For this review, take the finished solid that the model builds, in its own axes (mm). Round coordinates to 2 decimals unless told otherwise and drop trailing zeros. Order: outer loops, then holes, each group sorted by start corner. A loop starts at its lowest first (then second) coordinate and runs counter-clockwise, first axis right, second up.
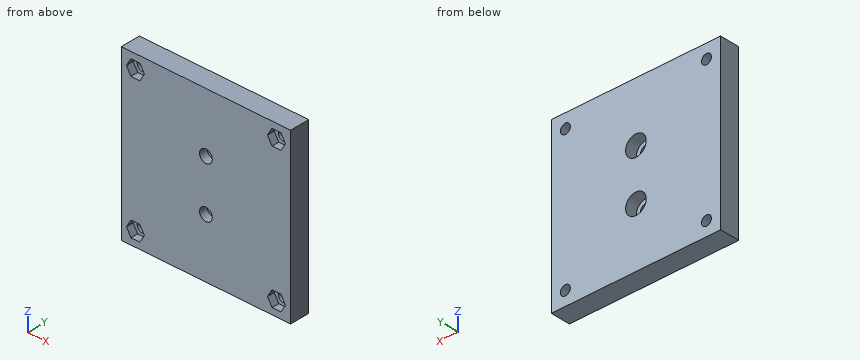
```python
from build123d import *

# Parameters (mm, degrees)
SKETCH_2_W          = 60
SKETCH_2_H          = 60
EXTRUDE_1_DEPTH     = 7
CUT_EXTRUDE_1_DEPTH = 2.6
CUT_EXTRUDE_2_REACH = 9
SKETCH_4_R          = 1.75
SKETCH_5_R          = 3.65
CUT_EXTRUDE_3_DEPTH = 4.1
CUT_EXTRUDE_4_REACH = 4.9
SKETCH_6_R          = 2.25


with BuildPart() as part:
    # 草圖2 → 填料-伸長1 (new body)
    with BuildSketch(Plane(origin=(0, 0, 0), x_dir=(1, 0, 0), z_dir=(0, 1, 0))):
        Rectangle(SKETCH_2_W, SKETCH_2_H)
    extrude(amount=EXTRUDE_1_DEPTH)

    # 草圖3 → 除料-伸長1 (cut)
    with BuildSketch(Plane.XZ):
        Polygon((-21.824573519, 25), (-23.41228676, 27.75), (-26.58771324, 27.75), (-28.175426481, 25), (-26.58771324, 22.25), (-23.41228676, 22.25), align=None)
        Polygon((23.41228676, 22.25), (21.824573519, 25), (23.41228676, 27.75), (26.58771324, 27.75), (28.175426481, 25), (26.58771324, 22.25), align=None)
        Polygon((21.824573519, -25), (23.41228676, -27.75), (26.58771324, -27.75), (28.175426481, -25), (26.58771324, -22.25), (23.41228676, -22.25), align=None)
        Polygon((-23.41228676, -22.25), (-21.824573519, -25), (-23.41228676, -27.75), (-26.58771324, -27.75), (-28.175426481, -25), (-26.58771324, -22.25), align=None)
    extrude(amount=-CUT_EXTRUDE_1_DEPTH, mode=Mode.SUBTRACT)

    # 草圖4 → 除料-伸長2 (cut, up to next)
    with BuildSketch(Plane(origin=(0, 7, 0), x_dir=(1, 0, 0), z_dir=(0, 1, 0)), mode=Mode.PRIVATE) as cut_extrude_2_sk1:
        with Locations((-25, 25)):
            Circle(SKETCH_4_R)
    cut_extrude_2_tool1 = extrude(cut_extrude_2_sk1.sketch, amount=-CUT_EXTRUDE_2_REACH, mode=Mode.PRIVATE) & part.part
    add(cut_extrude_2_tool1.solids().sort_by_distance((-25, 7, -25))[0], mode=Mode.SUBTRACT)
    # 草圖4 → 除料-伸長2 (cut, up to next)
    with BuildSketch(Plane(origin=(0, 7, 0), x_dir=(1, 0, 0), z_dir=(0, 1, 0)), mode=Mode.PRIVATE) as cut_extrude_2_sk2:
        with Locations((25, 25)):
            Circle(SKETCH_4_R)
    cut_extrude_2_tool2 = extrude(cut_extrude_2_sk2.sketch, amount=-CUT_EXTRUDE_2_REACH, mode=Mode.PRIVATE) & part.part
    add(cut_extrude_2_tool2.solids().sort_by_distance((25, 7, -25))[0], mode=Mode.SUBTRACT)
    # 草圖4 → 除料-伸長2 (cut, up to next)
    with BuildSketch(Plane(origin=(0, 7, 0), x_dir=(1, 0, 0), z_dir=(0, 1, 0)), mode=Mode.PRIVATE) as cut_extrude_2_sk3:
        with Locations((25, -25)):
            Circle(SKETCH_4_R)
    cut_extrude_2_tool3 = extrude(cut_extrude_2_sk3.sketch, amount=-CUT_EXTRUDE_2_REACH, mode=Mode.PRIVATE) & part.part
    add(cut_extrude_2_tool3.solids().sort_by_distance((25, 7, 25))[0], mode=Mode.SUBTRACT)
    # 草圖4 → 除料-伸長2 (cut, up to next)
    with BuildSketch(Plane(origin=(0, 7, 0), x_dir=(1, 0, 0), z_dir=(0, 1, 0)), mode=Mode.PRIVATE) as cut_extrude_2_sk4:
        with Locations((-25, -25)):
            Circle(SKETCH_4_R)
    cut_extrude_2_tool4 = extrude(cut_extrude_2_sk4.sketch, amount=-CUT_EXTRUDE_2_REACH, mode=Mode.PRIVATE) & part.part
    add(cut_extrude_2_tool4.solids().sort_by_distance((-25, 7, 25))[0], mode=Mode.SUBTRACT)

    # 草圖5 → 除料-伸長3 (cut)
    with BuildSketch(Plane(origin=(0, 7, 0), x_dir=(1, 0, 0), z_dir=(0, 1, 0))):
        with Locations((0, 9)):
            Circle(SKETCH_5_R)
        with Locations((0, -9)):
            Circle(SKETCH_5_R)
    extrude(amount=-CUT_EXTRUDE_3_DEPTH, mode=Mode.SUBTRACT)

    # 草圖6 → 除料-伸長4 (cut, up to next)
    with BuildSketch(Plane(origin=(0, 2.9, 0), x_dir=(1, 0, 0), z_dir=(0, 1, 0)), mode=Mode.PRIVATE) as cut_extrude_4_sk1:
        with Locations((0, 9)):
            Circle(SKETCH_6_R)
    cut_extrude_4_tool1 = extrude(cut_extrude_4_sk1.sketch, amount=-CUT_EXTRUDE_4_REACH, mode=Mode.PRIVATE) & part.part
    add(cut_extrude_4_tool1.solids().sort_by_distance((0, 2.9, -9))[0], mode=Mode.SUBTRACT)
    # 草圖6 → 除料-伸長4 (cut, up to next)
    with BuildSketch(Plane(origin=(0, 2.9, 0), x_dir=(1, 0, 0), z_dir=(0, 1, 0)), mode=Mode.PRIVATE) as cut_extrude_4_sk2:
        with Locations((0, -9)):
            Circle(SKETCH_6_R)
    cut_extrude_4_tool2 = extrude(cut_extrude_4_sk2.sketch, amount=-CUT_EXTRUDE_4_REACH, mode=Mode.PRIVATE) & part.part
    add(cut_extrude_4_tool2.solids().sort_by_distance((0, 2.9, 9))[0], mode=Mode.SUBTRACT)


solid = part.part
```
Q1. Take a section at C-C, the plane y = 4. State the section outline as (x, z) points, plus the area to 3 significant figures.
Q2. Take a section at B-B, the plane x = 0. State the section outline as (y, z) points.
Q3. Clearance check with flat-ended pins moving along their axes: pin 1 (3 mm diameter, centred on x = -25, z = -25.5, fed in from -Y); pin 2 (3 mm diameter, centred on x = 25, z = 25, fed in from +Y); pin 3 (6 mm diameter, centred on x = 0, z = 9, fed in from +Y). State where each tip first meets the part, or that it passes through.
Q4. Wall thickness on line 1 (Z direction, x = 0, y = 1.7); line 2 (X direction, y = 4.05, z = 25): over which ranges is each line inside the solid? List them lowest first.
Q5. Take a section at D-D, the plane x = -25. State the section outline as (y, z) points.
Q6. Take a section at A-A, the plane z = -9. State the section outline as (x, y) points.
Working result:
1. outline: (-30, -30) - (30, -30) - (30, 30) - (-30, 30) - close; hole circle Ø3.5 at (-25, -25); hole circle Ø3.5 at (-25, 25); hole circle Ø7.3 at (0, -9); hole circle Ø7.3 at (0, 9); hole circle Ø3.5 at (25, -25); hole circle Ø3.5 at (25, 25)
1. area: 3,480 mm2
2. outline: (0, -30) - (7, -30) - (7, -12.65) - (2.9, -12.65) - (2.9, -11.25) - (0, -11.25) - close; (0, -6.75) - (2.9, -6.75) - (2.9, -5.35) - (7, -5.35) - (7, 5.35) - (2.9, 5.35) - (2.9, 6.75) - (0, 6.75) - close; (0, 11.25) - (2.9, 11.25) - (2.9, 12.65) - (7, 12.65) - (7, 30) - (0, 30) - close
3. pin 1: stops at y = 2.6
3. pin 2: passes through
3. pin 3: stops at y = 2.9
4. line 1: z = -30 to -11.25, -6.75 to 6.75, 11.25 to 30
4. line 2: x = -30 to -26.75, -23.25 to 23.25, 26.75 to 30
5. outline: (0, -30) - (7, -30) - (7, -26.75) - (2.6, -26.75) - (2.6, -27.75) - (0, -27.75) - close; (0, -22.25) - (2.6, -22.25) - (2.6, -23.25) - (7, -23.25) - (7, 23.25) - (2.6, 23.25) - (2.6, 22.25) - (0, 22.25) - close; (0, 27.75) - (2.6, 27.75) - (2.6, 26.75) - (7, 26.75) - (7, 30) - (0, 30) - close
6. outline: (-30, 0) - (-2.25, 0) - (-2.25, 2.9) - (-3.65, 2.9) - (-3.65, 7) - (-30, 7) - close; (2.25, 0) - (30, 0) - (30, 7) - (3.65, 7) - (3.65, 2.9) - (2.25, 2.9) - close
